Could you check a few things on this model? Use its own coordinates, in mm. A direction names the side the tool comes from. Round coordinates to 2 decimals unless told otherwise and drop trailing zeros. Loops run counter-clockwise (first coordinate to the right, second up) from the corner with the lowest first, then second, coordinate; pieces in that order, holes last. Notation, with made-up numbers: (21, 7.25) -> (60, 7.25) arc R15 ccw to (60, 19.25) -> close; hole circle Ø1 at (28, -12.5). An arc over 180 degrees is marked (long way). One line per item, written item: value.
Autodesk Inventor part; units mm, degrees
ref_plane "YZ Plane" through (0, 0, 0) normal (1, 0, 0) x (0, 1, 0)
ref_plane "XZ Plane" through (0, 0, 0) normal (0, 1, 0) x (-1, 0, 0)
ref_plane "XY Plane" through (0, 0, 0) normal (0, 0, 1) x (1, 0, 0)
sketch "Sketch1" plane through (0, 0, 0) normal (1, 0, 0) x (0, 1, 0)
  line L0 (62.3549, 27.169) -> (-47.6451, 27.169)
  line L1 (-47.6451, 27.169) -> (-47.6451, -28.031)
  line L2 (-47.6451, -28.031) -> (62.3549, -28.031)
  line L3 (62.3549, -28.031) -> (62.3549, 27.169)
  point P0 (0, 0)
  dimension "d0" = 110
  dimension "d1" = 55.2
extrude "Extrusion1" add sketch "Sketch1" along normal blind 5
sketch "Sketch3" plane through (5, 0, 0) normal (1, 0, 0) x (0, 0, -1)
  line L0 (-27.169, -47.6451) -> (28.031, -47.6451)
  line L1 (28.031, -47.6451) -> (-4.969, -47.6451)
  line L2 (-4.969, -47.6451) -> (-4.969, -37.6451)
  point P0 (0, 0)
  dimension "d12" = 33
  dimension "d13" = 10
hole "Hole2" at (5, -37.6451, 4.969) direction (-1, 0, 0) diameter 3.2 end through all
sketch "Sketch13" plane through (5, 0, 0) normal (1, 0, 0) x (0, 0, -1)
  line L0 (-27.169, -47.6451) -> (28.031, -47.6451)
  line L1 (28.031, 62.3549) -> (-27.169, 62.3549)
  line L2 (28.031, -47.6451) -> (26.531, -47.6451)
  line L3 (26.531, -47.6451) -> (26.531, 62.3549)
  line L4 (26.531, 62.3549) -> (28.031, 62.3549)
  line L5 (28.031, 62.3549) -> (28.031, -47.6451)
  line L6 (-27.169, 62.3549) -> (-27.169, -47.6451)
  line L7 (28.031, 62.3549) -> (-27.169, 62.3549)
  line L8 (-27.169, -47.6451) -> (-25.669, -47.6451)
  line L9 (-25.669, -47.6451) -> (-25.669, 62.3549)
  line L10 (-25.669, 62.3549) -> (-27.169, 62.3549)
  line L11 (-27.169, 62.3549) -> (-27.169, -47.6451)
  line L12 (28.031, -47.6451) -> (-27.169, -47.6451)
  line L13 (-27.169, -47.6451) -> (-27.169, -45.6451)
  line L14 (-27.169, -45.6451) -> (28.031, -45.6451)
  line L15 (28.031, -45.6451) -> (28.031, -47.6451)
  point P0 (0, 0)
  point P1 (10.031, 62.3549)
  point P2 (-5.969, 62.3549)
  point P3 (26.531, -45.6451)
  point P4 (-25.669, -45.6451)
  point P5 (18.031, 62.3549)
  dimension "d42" = 1.5
  dimension "d43" = 1.5
  dimension "d44" = 2
extrude "Extrusion7" add sketch "Sketch13" along normal blind 6 contours L6 L14 L9 L0 | L9 L14 L3 L0 | L6 L1 L9 L14 | L3 L14 L5 L0 | L3 L1 L5 L14
sketch "Sketch14" plane through (0, 62.3549, 27.169) normal (0, 1, 0) x (1, 0, 0)
  line L0 (5, 1.5) -> (5, 53.7)
  line L1 (5, 53.7) -> (5, 38.7)
  line L2 (5, 1.5) -> (5, 16.5)
  line L3 (5, 38.7) -> (0, 38.7)
  line L4 (5, 21.7) -> (5, 38.7)
  line L5 (0, 55.2) -> (0, 0)
  line L6 (5, 38.7) -> (0, 38.7)
  line L7 (0, 38.7) -> (0, 16.5)
  line L8 (0, 16.5) -> (5, 16.5)
  line L9 (5, 16.5) -> (5, 38.7)
  point P0 (0, 27.169)
  dimension "d47" = 15
  dimension "d48" = 15
extrude "Extrusion8" add sketch "Sketch14" along normal blind 8.65
sketch "Sketch15" plane through (5, 0, 0) normal (1, 0, 0) x (0, 0, -1)
  line L0 (28.031, 62.3549) -> (11.531, 62.3549)
  line L1 (11.531, 62.3549) -> (4.531, 62.3549)
  line L2 (4.531, 62.3549) -> (4.531, 66.4495)
  line L3 (4.531, 66.4495) -> (11.531, 66.4495)
  line L4 (11.531, 66.4495) -> (11.531, 62.3549)
  line L5 (-10.669, 62.3549) -> (-25.669, 62.3549)
  line L6 (-10.669, 62.3549) -> (-3.669, 62.3549)
  line L7 (-3.669, 62.3549) -> (-3.669, 66.4495)
  line L8 (-3.669, 66.4495) -> (-10.669, 66.4495)
  line L9 (-10.669, 66.4495) -> (-10.669, 62.3549)
  point P0 (0, 0)
  dimension "d51" = 7
  dimension "d52" = 7
  dimension "d55" = 4.0946
extrude "Extrusion9" cut sketch "Sketch15" against normal blind 8.65
properties part number "pumpholderfinal"
(1) Imagine slicing it at B-B on y = 18.5. Write out the boundary of the cut face in (x, z).
Results below:
outline: (0, -28.03) -> (11, -28.03) -> (11, -26.53) -> (5, -26.53) -> (5, 25.67) -> (11, 25.67) -> (11, 27.17) -> (0, 27.17) -> close
(2) Imagine slicing it at A-A on x = 7.75. Write out the boundary of the cut face in (y, z), then the cut area to 3 significant figures.
Results below:
outline: (-47.65, -28.03) -> (62.35, -28.03) -> (62.35, -26.53) -> (-45.65, -26.53) -> (-45.65, 25.67) -> (62.35, 25.67) -> (62.35, 27.17) -> (-47.65, 27.17) -> close
area: 434 mm²
(3) We'd pull the mould along Z, two halves only. Please class faces 1 (the face through (8, 8, 25.669)), 2 (the face through (3, 64, 3.669)), 3 (the face through (3, 66.45, -8)), 4 (the face through (3, 69, -11.531)): +Z half, -Z half, draft (parallel to the pull), parting line (faces both ways), or undercut.
Results below:
face 1: undercut
face 2: +Z half
face 3: draft
face 4: -Z half
(4) For pin 1 Ø6.5 at (x, z) = (7, -6) entering from +Y; pin 2 Ø1.2 at (x, y) = (1.5, 64.5) entering from -Z; pin 3 Ø2 at (y, z) = (-18.5, -16) entering from +X; pin 4 Ø3.5 at (x, y) = (2, 70) entering from +Z, each with a flat end and sliding along its axis, tell me the tip position at first contact or that it passes through.
Results below:
pin 1: stops at y = 71
pin 2: stops at z = -4.53
pin 3: stops at x = 5
pin 4: stops at z = 10.67
(5) Imagine slicing it at C-C on z = -23. Write out the boundary of the cut face in (x, y), then the cut area to 3 significant figures.
Results below:
outline: (0, -47.65) -> (11, -47.65) -> (11, -45.65) -> (5, -45.65) -> (5, 62.35) -> (0, 62.35) -> close
area: 562 mm²
(6) Please list where these lines run through material, in increasing order: L1, parallel to Z at x = 9.5, y = 21.5; L2, parallel to Y at x = 0.75, z = -8; L3, parallel to Y at x = 2.5, z = 17.
Results below:
L1: z = -28.03 to -26.53, 25.67 to 27.17
L2: y = -47.65 to 62.35, 66.45 to 71
L3: y = -47.65 to 62.35
(7) On a 3-axis mill with a long thin cutter (end or side, diameter ignored), from which of +Z, -Z, +X, -X, +Y, -Y can I reach the whole of each face in a straight line? I mean faces 5 (the face through (3, 66.45, 7)), 6 (the face through (2, 69, 10.669)), 7 (the face through (3, 62.355, -16)), 8 (the face through (5, 12, 0)). Say none if no direction works.
Results below:
face 5: +Z, +X, -X
face 6: +Z, +X, -X, +Y
face 7: -Z, +X, -X
face 8: +X, +Y
(8) Imagine slicing it at D-D on z = -3. Write out the boundary of the cut face in (x, y).
Results below:
outline: (0, -47.65) -> (11, -47.65) -> (11, -45.65) -> (5, -45.65) -> (5, 71) -> (0, 71) -> close
